```python
from build123d import *

# Parameters (mm, degrees)
SKETCH1_R           = 1.5
BOSS_EXTRUDE1_DEPTH = 3


with BuildPart() as part:
    # Sketch1 → Boss-Extrude1 (new body)
    with BuildSketch(Plane(origin=(0, 0, 0), x_dir=(0, 0, -1), z_dir=(1, 0, 0))):
        with BuildLine():
            Line((-0.5, -3), (0.5, -3))
            ThreePointArc((0.5, -3), (2.708238703, -2.030685064), (3.489491568, 0.250878781))
            Line((3.489491568, 0.250878781), (3.489491568, 34.250878781))
            ThreePointArc((3.489491568, 34.250878781), (2.708238703, 36.532442626), (0.5, 37.501757562))
            Line((0.5, 37.501757562), (-0.5, 37.501757562))
            ThreePointArc((-0.5, 37.501757562), (-2.708238703, 36.532442626), (-3.489491568, 34.250878781))
            Line((-3.489491568, 34.250878781), (-3.489491568, 0.250878781))
            ThreePointArc((-3.489491568, 0.250878781), (-2.708238703, -2.030685064), (-0.5, -3))
        make_face()
        Circle(SKETCH1_R, mode=Mode.SUBTRACT)
        with Locations(Location((0, 34.501757562, 0), (0, 0, 180))):
            Circle(SKETCH1_R, mode=Mode.SUBTRACT)
    extrude(amount=BOSS_EXTRUDE1_DEPTH)


solid = part.part
```
Work out the finished part from the listing and answer in its coordinate system (mm). Round coordinates to 2 decimals unless told otherwise and drop trailing zeros. Write each loop counter-clockwise with the first axis right and the second up, starting at its lowest first coordinate (ties: lowest second). Pieces come first, ordered by that corner, then holes. Notation, with made-up numbers: (-9, 83.25) - (20, 83.25) arc R13 ccw to (20, 97.25) - close; hole circle Ø7 at (4.25, -2.75). An arc over 180 degrees is marked (long way). Return JSON: item names as keys, results as strings. Group by question number.
Q1. The part is cut by section C-C on z = 2.5. Write down the section's boundary in (x, y), then the cut area to 3 significant figures.
Q2. Each of these flat-tipped pins is pushed along its axis until it touches: pin 1 Ø1.5 at (x, y) = (1, 23.5) entering from +Z; pin 2 Ø1.5 at (x, y) = (1, 19) entering from -Z. Where does it stop, or does it pass through?
Q3. The mould has two halves that part along Z. Classify faces 1 (the cylindrical face through (1, 36, 0)), 2 (the flat face through (1, 17, 3.489)), 3 (the flat face through (1, 37.502, 0)), 4 (the flat face through (1, 17, -3.489)): released by +Z, released by -Z, zero draft, split by the parting line, or undercut.
Q4. Find the intervals of material crossed by L1, parallel to Y at x = 0.8, z = 0; L2, parallel to Z at x = 0.6, y = 20; L3, parallel to Z at x = 2.3, y = -1, in increasing order.
Q5. The part is cut by section A-A on z = 0. Write down the section's boundary in (x, y), then the cut area to 3 significant figures.
Q6. The part is cut by section B-B on x = 0.9. Write down the section's boundary in (y, z).
Q7. The part is cut by section D-D on z = -2. Write down the section's boundary in (x, y), then the cut area to 3 significant figures.
Solved:
{
 "1": {"outline": "(0, -2.24) - (3, -2.24) - (3, 36.74) - (0, 36.74) - close", "area": "117 mm²"},
 "2": {"pin 1": "z = 3.49", "pin 2": "z = -3.49"},
 "3": {"face 1": "undercut", "face 2": "released by +Z", "face 3": "zero draft", "face 4": "released by -Z"},
 "4": {"L1": "-3 to -1.5, 1.5 to 33, 36 to 37.5", "L2": "-3.49 to 3.49", "L3": "-3.33 to -1.12, 1.12 to 3.33"},
 "5": {"outline": "(0, -3) - (3, -3) - (3, -1.5) - (0, -1.5) - close; (0, 1.5) - (3, 1.5) - (3, 33) - (0, 33) - close; (0, 36) - (3, 36) - (3, 37.5) - (0, 37.5) - close", "area": "104 mm²"},
 "6": {"outline": "(-3, -0.5) arc R3 ccw to (0.25, -3.49) - (34.25, -3.49) arc R3 ccw to (37.5, -0.5) - (37.5, 0.5) arc R3 ccw to (34.25, 3.49) - (0.25, 3.49) arc R3 ccw to (-3, 0.5) - close; hole circle Ø3 at (0, 0); hole circle Ø3 at (34.5, 0)"},
 "7": {"outline": "(0, -2.6) - (3, -2.6) - (3, 37.1) - (0, 37.1) - close", "area": "119 mm²"}
}
